Source: three-view drawing plus pictorial views. Frame: mm from the lowest corner of the part. Give positions to 0.01 mm unless a question says otherwise; leave off trailing zeros. Order: outer loops, then holes, each group sorted by start corner. A loop starts at its lowest first (then second) coordinate and runs counter-clockwise, first axis right, second up. Notation, with made-up numbers: (-18, 22.25) - (18, 22.25) arc R16 cw to (18, 43.25) - close; hole circle Ø9 at (65.5, 85.25). An arc over 180 degrees is marked (long way). Use one line per item in the form item = value.
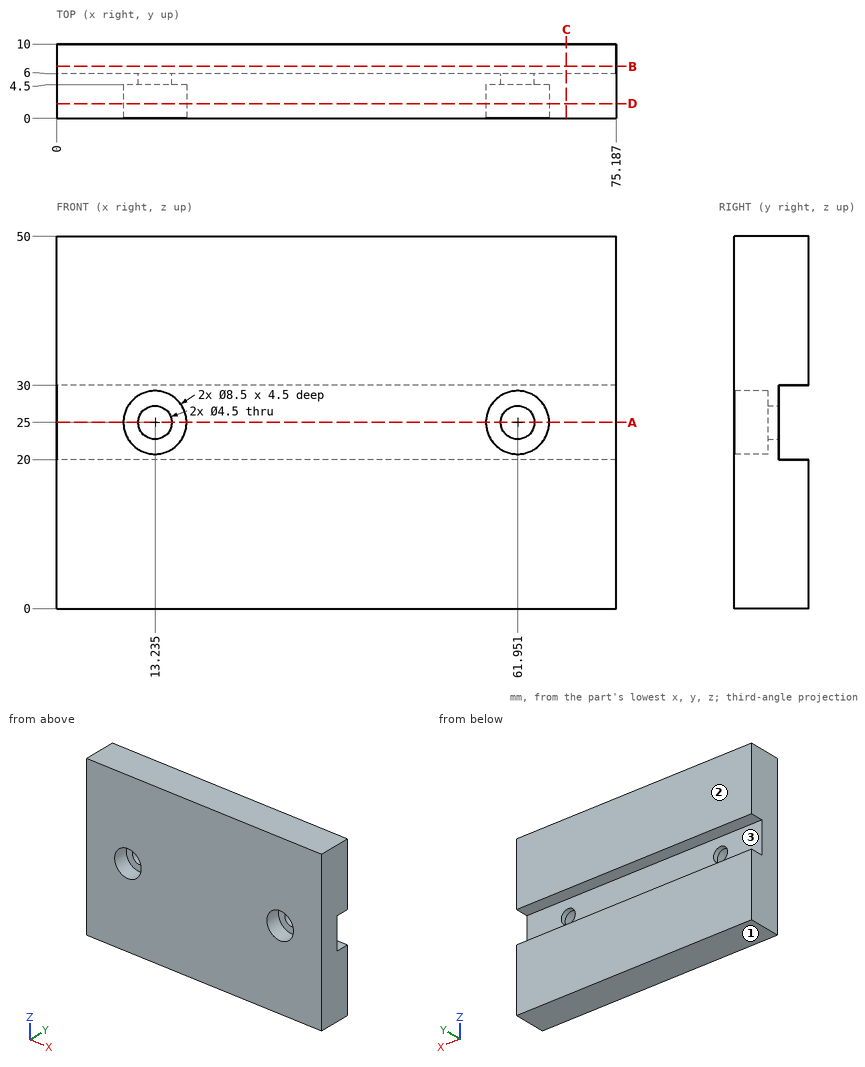
(1) Cut plane D-D on y = 2. Give the number of separate pieces and of enclosed holes in the cut face, plus the area to 3 significant figures.
Computed values:
separate_pieces = 1
enclosed_holes = 2
area = 3,650 mm²
(2) Cut plane B-B on y = 7. Output: boundary loops of the cut face in (x, z), plus the area to 3 significant figures.
Computed values:
outline = (0, 0) - (75.19, 0) - (75.19, 20) - (0, 20) - close; (0, 30) - (75.19, 30) - (75.19, 50) - (0, 50) - close
area = 3,010 mm²
(3) Cut plane A-A on z = 25. Output: boundary loops of the cut face in (x, y) (1 decimal).
Computed values:
outline = (0, 0) - (9, 0) - (9, 4.5) - (11, 4.5) - (11, 6) - (0, 6) - close; (15.5, 4.5) - (17.5, 4.5) - (17.5, 0) - (57.7, 0) - (57.7, 4.5) - (59.7, 4.5) - (59.7, 6) - (15.5, 6) - close; (64.2, 4.5) - (66.2, 4.5) - (66.2, 0) - (75.2, 0) - (75.2, 6) - (64.2, 6) - close
(4) Ray query, line 1 along Z through (x, y) = (27, 8); line 2 along Y through (x, z) = (57, 23). Return the intervals inside material, ascending.
Computed values:
line_1 = 0 to 20, 30 to 50
line_2 = 0 to 6
(5) Pull-direction query (Z, two-part tool) for the marked faces 1, 2 and 3; classes: released by +Z, released by -Z, zero draft, split by the parting line, or undercut.
Computed values:
face_1 = released by -Z
face_2 = zero draft
face_3 = undercut
(6) Contact query for flat-ended pins moving along their axis: pin 1 Ø11 at (x, z) = (36.5, 25) entering from +Y; pin 2 Ø4 at (x, z) = (13, 26.5) entering from -Y. Output: stop coordinate, or through.
Computed values:
pin_1 = 10
pin_2 = 4.5
(7) Cut plane C-C on x = 68.5. Output: boundary loops of the cut face in (y, z), plus the area to 3 significant figures.
Computed values:
outline = (0, 0) - (10, 0) - (10, 20) - (6, 20) - (6, 30) - (10, 30) - (10, 50) - (0, 50) - close
area = 460 mm²
